from build123d import *

# Parameters (mm, degrees)
SKETCH_1_W                        = 200
SKETCH_1_H                        = 20
SM_BASE_FLANGE_1_DEPTH            = 2
SM_EDGE_FLANGE_1_STRIP_W          = 13.4732
SM_EDGE_FLANGE_1_STRIP_H          = 2
SM_EDGE_FLANGE_1_STRIP_CUT_DEPTH  = 20
SM_EDGE_FLANGE_1_RELIEF_W         = 14.4732
SM_EDGE_FLANGE_1_RELIEF_H         = 1
SM_EDGE_FLANGE_1_RELIEF_CUT_DEPTH = 2
SM_EDGE_FLANGE_1_DEPTH            = 20
SKETCH_10_R                       = 2.75
CUT_EXTRUDE_2_DEPTH               = 10
SKETCH_11_R                       = 2.75
SKETCH_11_R_2                     = 1.75
CUT_EXTRUDE_3_DEPTH               = 10


# Sheet-metal steps are written as plain solids
with BuildPart() as part:
    # Sketch 1 → 基体-法兰1 (new body)
    with BuildSketch(Plane.XY):
        with Locations((0, -10)):
            Rectangle(SKETCH_1_W, SKETCH_1_H)
    extrude(amount=-SM_BASE_FLANGE_1_DEPTH)

    # 边线-法兰1 strip (across the edge) → 边线-法兰1 strip cut (cut)
    with BuildSketch(Plane(origin=(-100, -20, 0), x_dir=(0, 1, 0), z_dir=(1, 0, 0))):
        with Locations((-2, -1)):
            Rectangle(SM_EDGE_FLANGE_1_STRIP_W, SM_EDGE_FLANGE_1_STRIP_H)
    sm_edge_flange_1_strip_cut = extrude(amount=SM_EDGE_FLANGE_1_STRIP_CUT_DEPTH, mode=Mode.SUBTRACT)

    # 边线-法兰1 relief (on the sheet) → 边线-法兰1 relief cut (cut)
    with BuildSketch(Plane(origin=(-100, -15.2634, 0), x_dir=(0, 1, 0), z_dir=(0, 0, 1))):
        with Locations((-6.2366, -20.5)):
            Rectangle(SM_EDGE_FLANGE_1_RELIEF_W, SM_EDGE_FLANGE_1_RELIEF_H)
    sm_edge_flange_1_relief_cut = extrude(amount=-SM_EDGE_FLANGE_1_RELIEF_CUT_DEPTH, mode=Mode.SUBTRACT)

    # 边线-法兰1 section (across the edge) → 边线-法兰1 (add)
    with BuildSketch(Plane(origin=(-100, -20, 0), x_dir=(0, 1, 0), z_dir=(1, 0, 0))):
        with BuildLine():
            Line((0, 2.7366), (0, 20))
            Line((0, 20), (2, 20))
            Line((2, 20), (2, 2.7366))
            ThreePointArc((2, 2.7366), (2.801531583, 0.801531583), (4.7366, 0))
            Line((4.7366, 0), (4.7366, -2))
            ThreePointArc((4.7366, -2), (1.38731802, -0.61268198), (0, 2.7366))
        make_face()
    sm_edge_flange_1 = extrude(amount=SM_EDGE_FLANGE_1_DEPTH)

    # 草图10 → 切除-拉伸2 (cut)
    with BuildSketch(Plane(origin=(0, -18, 0), x_dir=(1, 0, 0), z_dir=(0, 1, 0))):
        with Locations(Location((-90, -10, 0), (0, 0, 270))):
            Circle(SKETCH_10_R)
    cut_extrude_2 = extrude(amount=-CUT_EXTRUDE_2_DEPTH, mode=Mode.SUBTRACT)

    # 镜向1: 边线-法兰1 strip cut, 边线-法兰1 relief cut, 边线-法兰1, 切除-拉伸2 across plane
    add(sm_edge_flange_1_strip_cut.mirror(Plane(origin=(0, 0, 0), x_dir=(0, 0, 1), z_dir=(1, 0, 0))), mode=Mode.SUBTRACT)
    add(sm_edge_flange_1_relief_cut.mirror(Plane(origin=(0, 0, 0), x_dir=(0, 0, 1), z_dir=(1, 0, 0))), mode=Mode.SUBTRACT)
    add(sm_edge_flange_1.mirror(Plane(origin=(0, 0, 0), x_dir=(0, 0, 1), z_dir=(1, 0, 0))))
    add(cut_extrude_2.mirror(Plane(origin=(0, 0, 0), x_dir=(0, 0, 1), z_dir=(1, 0, 0))), mode=Mode.SUBTRACT)

    # 草图11 → 切除-拉伸3 (cut)
    with BuildSketch(Plane(origin=(0, 0, -2), x_dir=(-1, 0, 0), z_dir=(0, 0, -1))):
        with Locations((0, -10)):
            Circle(SKETCH_11_R)
        with Locations((-11, -10)):
            Circle(SKETCH_11_R)
        with Locations(Location((11, -10, 0), (0, 0, 180))):
            Circle(SKETCH_11_R)
        with Locations((-60, -10)):
            Circle(SKETCH_11_R_2)
        with Locations((-50, -10)):
            Circle(SKETCH_11_R_2)
        with Locations(Location((60, -10, 0), (0, 0, 180))):
            Circle(SKETCH_11_R_2)
        with Locations(Location((50, -10, 0), (0, 0, 180))):
            Circle(SKETCH_11_R_2)
    extrude(amount=-CUT_EXTRUDE_3_DEPTH, mode=Mode.SUBTRACT)


solid = part.part
Work out the finished part from the listing and answer in its coordinate system (mm). A direction names the side the tool comes from. Give positions to 0.01 mm unless a question says otherwise; leave off trailing zeros. Order: outer loops, then holes, each group sorted by start corner. A loop starts at its lowest first (then second) coordinate and runs counter-clockwise, first axis right, second up. Notation, with made-up numbers: M -22,50 L 10,50 A18 cw 10,68 Z; hole C 59,-23 d7. An arc over 180 degrees is marked long. Return JSON: item names as keys, results as strings.
Q1. The mould has two halves that part along Z. Classify faces 1 (the face through (-48.331, -10.526, -1.014)), 2 (the face through (-90.14, -18.576, -0.649)), 3 (the face through (92.44, -18.99, 11.27)): pulls with the +Z half, pulls with the -Z half, needs draft (parallel to the pull), parting line crosses it, or undercut.
Answer below:
{"face 1": "needs draft", "face 2": "pulls with the -Z half", "face 3": "undercut"}
Q2. Find section A-A, the plane z = 10. Write down the section's boundary in (x, y).
Answer below:
{"outline": "M -100,-20 L -92.75,-20 L -92.75,-18 L -100,-18 Z; M -87.25,-20 L -80,-20 L -80,-18 L -87.25,-18 Z; M 80,-20 L 87.25,-20 L 87.25,-18 L 80,-18 Z; M 92.75,-20 L 100,-20 L 100,-18 L 92.75,-18 Z"}
Q3. Find the intervals of material crossed by line 1 along X through (y, z) = (-19.2, 10); line 2 along Y through (x, z) = (50, -0.75); line 3 along Y through (x, z) = (11, -1.15), in increasing order. Write a range as [from, to].
Answer below:
{"line 1": "x = [-100, -92.75], [-87.25, -80], [80, 87.25], [92.75, 100]", "line 2": "y = [-20, -11.75], [-8.25, 0]", "line 3": "y = [-20, -12.75], [-7.25, 0]"}
Q4. Each of these flat-tipped pins is pushed along its axis until it touches: pin 1 (0.5 mm diameter, centred on x = 79.5, z = -0.5, fed in from -Y); pin 2 (7 mm diameter, centred on x = 11, y = -10, fed in from +Z); pin 3 (7 mm diameter, centred on x = 90, z = 10, fed in from -Y); pin 4 (8.5 mm diameter, centred on x = 94, z = 12, fed in from +Y). Where does it stop, or does it pass through?
Answer below:
{"pin 1": "stops at y = -14.26", "pin 2": "stops at z = 0", "pin 3": "stops at y = -20", "pin 4": "stops at y = -18"}
Q5. Find section B-B, the plane x = -90. Write down the section's boundary in (y, z).
Answer below:
{"outline": "M -20,2.74 A4.74 ccw -15.26,-2 L 0,-2 L 0,0 L -15.26,0 A2.74 cw -18,2.74 L -18,7.25 L -20,7.25 Z; M -20,12.75 L -18,12.75 L -18,20 L -20,20 Z"}
Q6. Find section C-C, the plane x = 60. Write down the section's boundary in (y, z).
Answer below:
{"outline": "M -20,-2 L -11.75,-2 L -11.75,0 L -20,0 Z; M -8.25,-2 L 0,-2 L 0,0 L -8.25,0 Z"}
Q7. Which of the six approach directions +Z, -Z, +X, -X, +Y, -Y give full straight-line access (tool end or side, diameter ignored) to faces 4 (the face through (-80, -18.4, 6.7)), 5 (the face through (90.14, -18.576, -0.649)), 6 (the face through (-1, -5, 0)), 7 (the face through (-90, -18, 13))?
Answer below:
{"face 4": "+Z, -Z, -Y", "face 5": "-Z, +X, -Y", "face 6": "+Z, +Y", "face 7": "+Z, +X, -X, +Y"}
Q8. Find section D-D, the plane y = -4.5. Write down the section's boundary in (x, z), and give its area (3 significant figures).
Answer below:
{"outline": "M -100,-2 L 100,-2 L 100,0 L -100,0 Z", "area": "400 mm^2"}
